Input: part model. Units: mm. Frame: model coordinates. A direction names the side the tool comes from. Coordinates: 2 decimals unless noted, no trailing zeros. Loops run counter-clockwise (first coordinate to the right, second up) from the corner with the lowest first, then second, coordinate; pieces in that order, holes last.
(1) Line query: L1, parallel to Y at x = 9.5, z = 6; L2, parallel to Z at x = -13, y = 10.5; L3, parallel to Y at x = -12, z = 6. Output: solid intervals per line, ascending.
(2) Section C-C, the plane z = 3.75. Return loops of the section in (x, y), then the cut area to 3 significant figures.
(3) Section D-D, the plane x = 8. Return loops of the section in (y, z), then the cut area to 3 significant figures.
(4) Contact query for flat-ended pins moving along their axis: P1, Ø3, axis at x = 6.5, z = 4, coming from the -Y side; P2, Ø12, axis at x = 2, y = -5.5, coming from the -Z side; P3, Ø1, axis at y = 5.5, z = 7.5, coming from the +X side; P4, Ø2, axis at x = 0, y = -12.5, coming from the -Z side. Output: stop coordinate, or through.
(5) Mould query, pull axis X, two halves, no side actions, for faces 1 (the face through (1.172, 8.923, 6.162)), 2 (the face through (-13.887, -10.648, 6.923)), 3 (the face through (8, -8, 12.5)). Classes: released by +X, released by -X, zero draft, split by the parting line, or undercut.
(6) Set-up query: faces 4 (the face through (0.228, 14.235, 6.162)), 5 (the face through (6.691, -12.864, 0.74)). Return all of +Z, -Z, +X, -X, +Y, -Y with unobstructed straight access to the full face (end or side cutting, diameter ignored); none if empty.
(7) Section B-B, the plane x = 0. Return loops of the section in (y, z), then the cut area to 3 significant figures.
(8) Section A-A, the plane y = 0. Return loops of the section in (x, z), then the cut area to 4 significant figures.
```python
from build123d import *

# Parameters (mm, degrees)
SKETCH_1_R          = 14.5
EXTRUDE_1_DEPTH     = 1.5
SKETCH_2_R          = 17.5
EXTRUDE_2_DEPTH     = 11
SKETCH_3_R          = 1.75
SKETCH_3_R_2        = 9
CUT_EXTRUDE_1_DEPTH = 26.5


with BuildPart() as part:
    # 草图1 → 凸台-拉伸1 (new body)
    with BuildSketch(Plane.XY):
        Circle(SKETCH_1_R)
    extrude(amount=EXTRUDE_1_DEPTH)

    # 草图2 → 凸台-拉伸2 (add)
    with BuildSketch(Plane.XY.offset(1.5)):
        Circle(SKETCH_2_R)
    extrude(amount=EXTRUDE_2_DEPTH)

    # 草图3 → 切除-拉伸1 (cut)
    with BuildSketch(Plane(origin=(0, 0, 0), x_dir=(-1, 0, 0), z_dir=(0, 0, -1))):
        with Locations((0, 12.5)):
            Circle(SKETCH_3_R)
        Circle(SKETCH_3_R_2)
        with Locations((10.825317547, 6.25)):
            Circle(SKETCH_3_R)
        with Locations((10.825317547, -6.25)):
            Circle(SKETCH_3_R)
        with Locations((0, -12.5)):
            Circle(SKETCH_3_R)
        with Locations((-10.825317547, -6.25)):
            Circle(SKETCH_3_R)
        with Locations((-10.825317547, 6.25)):
            Circle(SKETCH_3_R)
    extrude(amount=-CUT_EXTRUDE_1_DEPTH, mode=Mode.SUBTRACT)


solid = part.part
```
Report:
1. L1: y = -14.7 to -7.39, -5.11 to 5.11, 7.39 to 14.7
1. L2: z = 1.5 to 12.5
1. L3: y = -12.74 to -7.55, -4.95 to 4.95, 7.55 to 12.74
2. outline: circle Ø35 at (0, 0); hole circle Ø3.5 at (-10.83, -6.25); hole circle Ø3.5 at (-10.83, 6.25); hole circle Ø18 at (0, 0); hole circle Ø3.5 at (0, -12.5); hole circle Ø3.5 at (0, 12.5); hole circle Ø3.5 at (10.83, -6.25); hole circle Ø3.5 at (10.83, 6.25)
2. area: 650 mm2
3. outline: (-15.56, 1.5) - (-12.09, 1.5) - (-12.09, 0) - (-4.12, 0) - (-4.12, 12.5) - (-15.56, 12.5) - close; (4.12, 0) - (12.09, 0) - (12.09, 1.5) - (15.56, 1.5) - (15.56, 12.5) - (4.12, 12.5) - close
3. area: 276 mm2
4. P1: stops at y = -16.77
4. P2: stops at z = 0
4. P3: stops at x = 16.77
4. P4: passes through
5. face 1: undercut
5. face 2: split by the parting line
5. face 3: zero draft
6. face 4: +Z, -Z
6. face 5: -Z
7. outline: (-17.5, 1.5) - (-14.5, 1.5) - (-14.5, 0) - (-14.25, 0) - (-14.25, 12.5) - (-17.5, 12.5) - close; (-10.75, 0) - (-9, 0) - (-9, 12.5) - (-10.75, 12.5) - close; (9, 0) - (10.75, 0) - (10.75, 12.5) - (9, 12.5) - close; (14.25, 0) - (14.5, 0) - (14.5, 1.5) - (17.5, 1.5) - (17.5, 12.5) - (14.25, 12.5) - close
7. area: 116 mm2
8. outline: (-17.5, 1.5) - (-14.5, 1.5) - (-14.5, 0) - (-9, 0) - (-9, 12.5) - (-17.5, 12.5) - close; (9, 0) - (14.5, 0) - (14.5, 1.5) - (17.5, 1.5) - (17.5, 12.5) - (9, 12.5) - close
8. area: 203.5 mm2
